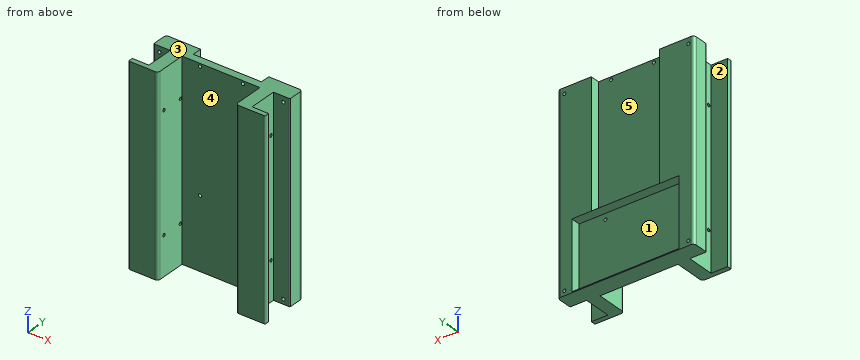
from build123d import *

# Parameters (mm, degrees)
EXTRUDE_2_DEPTH          = 100
SKETCH_4_W               = 110.09382566
SKETCH_4_H               = 70
SKETCH_4_W_2             = 70
SKETCH_4_H_2             = 129.351240965
CUT_EXTRUDE_1_DEPTH      = 10
SKETCH_5_R               = 1.6
CUT_EXTRUDE_2_DEPTH      = 22
SKETCH_6_W               = 17
SKETCH_6_H               = 28.6
CUT_EXTRUDE_3_DEPTH      = 101
CUT_EXTRUDE_3_DEPTH_BACK = 101
SKETCH_7_R               = 1.6
CUT_EXTRUDE_4_DEPTH      = 84.5
FILLET_1_R               = 1
FILLET_2_R               = 3


with BuildPart() as part:
    # 草图1 → 凸台-拉伸2 (new body, symmetric)
    with BuildSketch(Plane.XY):
        Polygon((-40.540540541, -50.17722933), (-40.540540541, -17.800330782), (39.459459459, -17.800330782), (39.459459459, -50.17722933), (69.459459459, -50.17722933), (69.459459459, -0.17722933), (-70.540540541, -0.17722933), (-70.540540541, -50.17722933), align=None)
    extrude(amount=EXTRUDE_2_DEPTH, both=True)

    # 草图4 → 切除-拉伸1 (cut)
    with BuildSketch(Plane(origin=(0, 0, 0), x_dir=(1, 0, 0), z_dir=(0, 1, 0))):
        with Locations((-0.04691283, 64.024061656)):
            Rectangle(SKETCH_4_W, SKETCH_4_H)
        with Locations((0, -35.675620483)):
            Rectangle(SKETCH_4_W_2, SKETCH_4_H_2)
    extrude(amount=-CUT_EXTRUDE_1_DEPTH, mode=Mode.SUBTRACT)

    # 草图5 → 切除-拉伸2 (cut)
    with BuildSketch(Plane(origin=(0, 0, 0), x_dir=(1, 0, 0), z_dir=(0, 1, 0))):
        with Locations((29, 96)):
            Circle(SKETCH_5_R)
        with Locations((-50, 53)):
            Circle(SKETCH_5_R)
        with Locations((28, 35)):
            Circle(SKETCH_5_R)
        with Locations((-50, 90)):
            Circle(SKETCH_5_R)
        with Locations((-22, 27)):
            Circle(SKETCH_5_R)
        with Locations((22, 27)):
            Circle(SKETCH_5_R)
        with Locations((-22, -97)):
            Circle(SKETCH_5_R)
        with Locations((22, -97)):
            Circle(SKETCH_5_R)
        with Locations((-64.69341522, 95.162832005)):
            Circle(SKETCH_5_R)
        with Locations((62.668909511, 95.162832005)):
            Circle(SKETCH_5_R)
        with Locations((62.668909511, -94.06900635)):
            Circle(SKETCH_5_R)
        with Locations((-64.69341522, -94.06900635)):
            Circle(SKETCH_5_R)
    extrude(amount=-CUT_EXTRUDE_2_DEPTH, mode=Mode.SUBTRACT)

    # 草图6 → 切除-拉伸3 (cut, two sides)
    with BuildSketch(Plane.XY) as cut_extrude_3_sk:
        with Locations((-62.040540541, -30.993677516)):
            Rectangle(SKETCH_6_W, SKETCH_6_H)
        with Locations((60.959459459, -30.993677516)):
            Rectangle(SKETCH_6_W, SKETCH_6_H)
    extrude(amount=CUT_EXTRUDE_3_DEPTH, mode=Mode.SUBTRACT)
    extrude(cut_extrude_3_sk.sketch, amount=-CUT_EXTRUDE_3_DEPTH_BACK, mode=Mode.SUBTRACT)

    # 草图7 → 切除-拉伸4 (cut, symmetric)
    with BuildSketch(Plane(origin=(0, 0, 0), x_dir=(0, 0, -1), z_dir=(1, 0, 0))):
        with Locations((-60, -20)):
            Circle(SKETCH_7_R)
        with Locations((-60, -42)):
            Circle(SKETCH_7_R)
        with Locations((60, -42)):
            Circle(SKETCH_7_R)
        with Locations((60, -20)):
            Circle(SKETCH_7_R)
    extrude(amount=CUT_EXTRUDE_4_DEPTH, both=True, mode=Mode.SUBTRACT)

    # 圆角1
    fillet_1_edges = [part.edges().sort_by_distance(p)[0] for p in [
        (-70.540540541, -16.693677516, 0),
        (69.459459459, -16.693677516, 0),
        (69.459459459, -50.17722933, 0),
        (-70.540540541, -50.17722933, 0),
    ]]
    fillet(fillet_1_edges, radius=FILLET_1_R)

    # 圆角2
    fillet_2_edges = [part.edges().sort_by_distance(p)[0] for p in [
        (-70.540540541, -0.17722933, 0),
        (69.459459459, -0.17722933, 0),
        (39.459459459, -50.17722933, 0),
        (-40.540540541, -50.17722933, 0),
    ]]
    fillet(fillet_2_edges, radius=FILLET_2_R)


solid = part.part
Verification items for the finished model (mm, model axes). Face numbers are marked on the shaded views. A direction names the side the tool comes from. Coordinates: 2 decimals unless noted, no trailing zeros. Loops run counter-clockwise (first coordinate to the right, second up) from the corner with the lowest first, then second, coordinate; pieces in that order, holes last. Notation, with made-up numbers: (45.5, 44.5) -> (98.5, 44.5) arc R26 ccw to (98.5, 82.5) -> close; hole circle Ø6 at (0, 7). An arc over 180 degrees is marked (long way). Write each question's results on one line, items separated by ' | '.
Item 1: Gauge pin test, flat ends, axial feed: pin 1 (1.5 mm diameter, centred on x = -4, z = -42.5, fed in from +Y); pin 2 (1.5 mm diameter, centred on x = 31, z = -40, fed in from -Y); pin 3 (2.5 mm diameter, centred on x = -64.69, z = 94.07, fed in from +Y). Record the tip position at first contact, or that the pin passes through.
Found:
pin 1: stops at y = -10 | pin 2: stops at y = -17.8 | pin 3: stops at y = -45.29
Item 2: Tool access check on the marked faces 3, 4 and 5. Record the directions out of +Z, -Z, +X, -X, +Y, -Y that give a thin tool (end or side, any length) a straight path to the whole face; none if there is none.
Found:
face 3: +Z, +X, -X, +Y, -Y | face 4: +Z, -Z, -Y | face 5: +Z, +Y
Item 3: Section check A-A, the plane x = 57.5. Enter the section's corners in (y, z), plus the area to 3 significant figures.
Found:
outline: (-50.18, -100) -> (-45.29, -100) -> (-45.29, 100) -> (-50.18, 100) -> close; (-16.69, -100) -> (-0.18, -100) -> (-0.18, 100) -> (-16.69, 100) -> close | area: 4,280 mm2
Item 4: Mould release check, pull along X, two halves, no side actions. Record for the marked faces 1 and 2: +X half, -X half, draft (parallel to the pull), parting line (faces both ways), or undercut.
Found:
face 1: undercut | face 2: draft
Item 5: Section check C-C, the plane z = -74. Enter the section's corners in (x, y).
Found:
outline: (-70.54, -49.18) arc R1 ccw to (-69.54, -50.18) -> (-43.54, -50.18) arc R3 ccw to (-40.54, -47.18) -> (-40.54, -17.8) -> (39.46, -17.8) -> (39.46, -47.18) arc R3 ccw to (42.46, -50.18) -> (68.46, -50.18) arc R1 ccw to (69.46, -49.18) -> (69.46, -45.29) -> (52.46, -45.29) -> (52.46, -16.69) -> (68.46, -16.69) arc R1 ccw to (69.46, -15.69) -> (69.46, -3.18) arc R3 ccw to (66.46, -0.18) -> (55, -0.18) -> (55, -10) -> (-55.09, -10) -> (-55.09, -0.18) -> (-67.54, -0.18) arc R3 ccw to (-70.54, -3.18) -> (-70.54, -15.69) arc R1 ccw to (-69.54, -16.69) -> (-53.54, -16.69) -> (-53.54, -45.29) -> (-70.54, -45.29) -> close
Item 6: Section check B-B, the plane y = -37.5. Enter the section's corners in (x, z), plus the area to 3 significant figures.
Found:
outline: (-53.54, -100) -> (-40.54, -100) -> (-40.54, 100) -> (-53.54, 100) -> close; (39.46, -100) -> (52.46, -100) -> (52.46, 100) -> (39.46, 100) -> close | area: 5,200 mm2
Item 7: Material ranges on L1, parallel to Y at x = 44, z = -60; L2, parallel to Z at x = 48, y = -42; L3, parallel to X at y = -18.5, z = -66.5, recorded low to high.
Found:
L1: y = -50.18 to -43.6, -40.4 to -21.6, -18.4 to -10 | L2: z = -100 to -61.6, -58.4 to 58.4, 61.6 to 100 | L3: x = -53.54 to -40.54, 39.46 to 52.46
